```python
from build123d import *

# Parameters (mm, degrees)
SKETCH1_R           = 6
BOSS_EXTRUDE1_DEPTH = 3


with BuildPart() as part:
    # Sketch1 → Boss-Extrude1 (new body)
    with BuildSketch(Plane(origin=(0, 0, 0), x_dir=(1, 0, 0), z_dir=(0, 1, 0))):
        with BuildLine():
            Line((-62.687563754, 15.857142857), (277.312436246, 15.857142857))
            ThreePointArc((277.312436246, 15.857142857), (287.312436246, 5.857142857), (277.312436246, -4.142857143))
            Line((277.312436246, -4.142857143), (-62.687563754, -4.142857143))
            ThreePointArc((-62.687563754, -4.142857143), (-72.687563754, 5.857142857), (-62.687563754, 15.857142857))
        make_face()
        with Locations((-62.687563754, 5.857142857)):
            Circle(SKETCH1_R, mode=Mode.SUBTRACT)
        with Locations((277.312436246, 5.857142857)):
            Circle(SKETCH1_R, mode=Mode.SUBTRACT)
        with Locations((107.312436246, 5.857142857)):
            Circle(SKETCH1_R, mode=Mode.SUBTRACT)
    extrude(amount=BOSS_EXTRUDE1_DEPTH)


solid = part.part
```
For this review, take the finished solid that the model builds, in its own axes (mm). Round coordinates to 2 decimals unless told otherwise and drop trailing zeros. Order: outer loops, then holes, each group sorted by start corner. A loop starts at its lowest first (then second) coordinate and runs counter-clockwise, first axis right, second up. Notation, with made-up numbers: (56, 51) -> (68, 51) arc R14 ccw to (68, 74) -> close; hole circle Ø11 at (30, 24). An arc over 180 degrees is marked (long way). Use a Markdown table: item, result.
Item 1: For pin 1 (11 mm diameter, centred on x = 277.31, z = -5.86, fed in from -Y); pin 2 (1 mm diameter, centred on x = 10, z = -3, fed in from -Y), all flat-tipped, find the tip position at first contact; note any pin that passes through.
Resolved:
| item | result |
|---|---|
| pin 1 | passes through |
| pin 2 | stops at y = 0 |
Item 2: Take a section at B-B (y = 0.45). State the section outline as (x, z) points, plus the area to 3 significant figures.
Resolved:
| item | result |
|---|---|
| outline | (-62.69, -15.86) -> (277.31, -15.86) arc R10 ccw to (277.31, 4.14) -> (-62.69, 4.14) arc R10 ccw to start; hole circle Ø12 at (-62.69, -5.86); hole circle Ø12 at (107.31, -5.86); hole circle Ø12 at (277.31, -5.86) |
| area | 6,770 mm² |
Item 3: Draft analysis for pull direction X (two halves, no side actions). For faces 1 (the cylindrical face through (287.31, 1.48, -6.08)), 2 (the flat face through (110, 3, -13)), 3 (the cylindrical face through (113.035, 1.479, -7.659)), state which applies: +X half, -X half, draft (parallel to the pull), parting line (faces both ways), or undercut.
Resolved:
| item | result |
|---|---|
| face 1 | +X half |
| face 2 | draft |
| face 3 | undercut |
Item 4: Take a section at A-A (z = -8.75). State the section outline as (x, y) points.
Resolved:
| item | result |
|---|---|
| outline | (-72.26, 0) -> (-67.94, 0) -> (-67.94, 3) -> (-72.26, 3) -> close; (-57.43, 0) -> (102.06, 0) -> (102.06, 3) -> (-57.43, 3) -> close; (112.57, 0) -> (272.06, 0) -> (272.06, 3) -> (112.57, 3) -> close; (282.57, 0) -> (286.88, 0) -> (286.88, 3) -> (282.57, 3) -> close |
Item 5: For line 1 along X through (y, z) = (1.9, -5.5); line 2 along X through (y, z) = (1.45, -10.25); line 3 along X through (y, z) = (0.45, -12.75), list the stretches that pass through material, from the lowest coordinate up. Write a range as [from, to].
Resolved:
| item | result |
|---|---|
| line 1 | x = [-72.68, -68.68], [-56.7, 101.32], [113.3, 271.32], [283.3, 287.31] |
| line 2 | x = [-71.67, -66.77], [-58.6, 103.23], [111.4, 273.23], [281.4, 286.3] |
| line 3 | x = [-69.93, 284.56] |
